Model file for the job. Use its own axes, mm. A direction names the side the tool comes from. Coordinates: 2 decimals unless noted, no trailing zeros. Order: outer loops, then holes, each group sorted by start corner. A loop starts at its lowest first (then second) coordinate and runs counter-clockwise, first axis right, second up. Notation, with made-up numbers: (49, 18) -> (72, 18) arc R9 cw to (72, 35) -> close; hole circle Ø11 at (-23.5, 2). An arc over 180 degrees is marked (long way). Return JSON: item names as keys, results as strings. Group by question number.
1) Cut at B-B (y = -8). Write the cut outline in (x, z), and give its area (3 significant figures).
2) Cut at C-C (x = 56). Write the cut outline in (y, z).
3) Probe line 1 (X direction, y = -12.5, z = -8.5); line 2 (Y direction, x = -24, z = 11.25); line 3 (Y direction, x = 71, z = 1.75). List the from-to ranges inside material, lowest first.
4) Pull direction Y, two halves, no side cores. Call faces 1 (the flat face through (-69, 0, 0)), 2 (the flat face through (73, -24.25, -2)), 3 (the flat face through (69, 0, 0)), 4 (the flat face through (77, 26.25, 0)): +Y half, -Y half, draft (parallel to the pull), parting line (faces both ways), or undercut.
5) Flat gauge pins, fed straight in: pin 1 (8.5 mm diameter, centred on x = 0, z = 4, fed in from -Y); pin 2 (2.5 mm diameter, centred on x = 73.5, y = -23, fed in from -Z); pin 3 (0.9 mm diameter, centred on x = 70.5, y = -22.5, fed in from +Z). Where does each tip first touch, or does it go through?
6) Which spindle directions (+Z, -Z, +X, -X, +Y, -Y) get a long thin tool onto all of the face, cutting with end or side? Do faces 5 (the flat face through (67, -23, -2)), 6 (the flat face through (73, -23, 0.666)), 7 (the flat face through (66, 24, 0)). Say none if no direction does.
7) Cut at A-A (z = -2.25). Write the cut outline in (x, y).
from build123d import *

# Parameters (mm, degrees)
SKETCH1_W                = 138
SKETCH1_H                = 42.5
BOSS_EXTRUDE1_DEPTH      = 14.5
BOSS_EXTRUDE2_DEPTH      = 20
BOSS_EXTRUDE2_DEPTH_BACK = 3
BOSS_EXTRUDE2_START      = 69
SKETCH2_W                = 15
SKETCH2_H                = 5
BOSS_EXTRUDE3_DEPTH      = 10
BOSS_EXTRUDE3_DEPTH_BACK = 2
BOSS_EXTRUDE3_START      = 69
SKETCH2_3_W              = 6
SKETCH2_3_H              = 3


with BuildPart() as part:
    # Sketch1 → Boss-Extrude1 (new, symmetric)
    with BuildSketch(Plane.XY):
        Rectangle(SKETCH1_W, SKETCH1_H)
    extrude(amount=BOSS_EXTRUDE1_DEPTH, both=True)

    # Sketch2 → Boss-Extrude2 (add, two sides: drawn at the far end of the back side and taken through both)
    with BuildSketch(Plane(origin=(0, 0, 0), x_dir=(0, 0, -1), z_dir=(1, 0, 0)).offset(BOSS_EXTRUDE2_START - BOSS_EXTRUDE2_DEPTH_BACK)):
        with Locations((0, 23.75)):
            Rectangle(SKETCH2_W, SKETCH2_H)
    extrude(amount=BOSS_EXTRUDE2_DEPTH + BOSS_EXTRUDE2_DEPTH_BACK)

    # Sketch2<3> → Boss-Extrude3 (add, two sides: drawn at the far end of the back side and taken through both)
    with BuildSketch(Plane(origin=(0, 0, 0), x_dir=(0, 0, -1), z_dir=(1, 0, 0)).offset(BOSS_EXTRUDE3_START - BOSS_EXTRUDE3_DEPTH_BACK)):
        with Locations((2.334145167, -22.75)):
            Rectangle(SKETCH2_3_W, SKETCH2_3_H)
    extrude(amount=BOSS_EXTRUDE3_DEPTH + BOSS_EXTRUDE3_DEPTH_BACK)


solid = part.part
Answers below:
{
 "1": {"outline": "(-69, -14.5) -> (69, -14.5) -> (69, 14.5) -> (-69, 14.5) -> close", "area": "4,000 mm^2"},
 "2": {"outline": "(-21.25, -14.5) -> (21.25, -14.5) -> (21.25, 14.5) -> (-21.25, 14.5) -> close"},
 "3": {"line 1": "x = -69 to 69", "line 2": "y = -21.25 to 21.25", "line 3": "y = 21.25 to 26.25"},
 "4": {"face 1": "draft", "face 2": "-Y half", "face 3": "undercut", "face 4": "+Y half"},
 "5": {"pin 1": "stops at y = -21.25", "pin 2": "stops at z = -5.33", "pin 3": "stops at z = 0.67"},
 "6": {"face 5": "+Z, -Z, -X, -Y", "face 6": "+Z, +X, -X, -Y", "face 7": "+Z, -Z, -X, +Y"},
 "7": {"outline": "(-69, -21.25) -> (67, -21.25) -> (67, -24.25) -> (79, -24.25) -> (79, -21.25) -> (69, -21.25) -> (69, 21.25) -> (89, 21.25) -> (89, 26.25) -> (66, 26.25) -> (66, 21.25) -> (-69, 21.25) -> close"}
}
